from build123d import *

# Parameters (mm, degrees)
SKETCH1_R           = 1.5
BOSS_EXTRUDE1_DEPTH = 1.35
CHAMFER1_SIZE       = 0.4


with BuildPart() as part:
    # Sketch1 → Boss-Extrude1 (new body, symmetric)
    with BuildSketch(Plane(origin=(0, 0, 0), x_dir=(1, 0, 0), z_dir=(0, 1, 0))):
        with BuildLine():
            Line((-13.25, 3.25), (13.25, 3.25))
            ThreePointArc((13.25, 3.25), (16.5, 0), (13.25, -3.25))
            Line((13.25, -3.25), (-13.25, -3.25))
            ThreePointArc((-13.25, -3.25), (-16.5, 0), (-13.25, 3.25))
        make_face()
        with Locations((-13.25, 0)):
            Circle(SKETCH1_R, mode=Mode.SUBTRACT)
        with Locations((13.25, 0)):
            Circle(SKETCH1_R, mode=Mode.SUBTRACT)
        Circle(SKETCH1_R, mode=Mode.SUBTRACT)
    extrude(amount=BOSS_EXTRUDE1_DEPTH, both=True)

    # Chamfer1
    chamfer1_edges = [part.edges().sort_by_distance(p)[0] for p in [
        (16.5, 1.35, 0),
        (0, 1.35, -3.25),
        (-16.5, 1.35, 0),
        (0, 1.35, 3.25),
    ]]
    chamfer(chamfer1_edges, length=CHAMFER1_SIZE)


solid = part.part
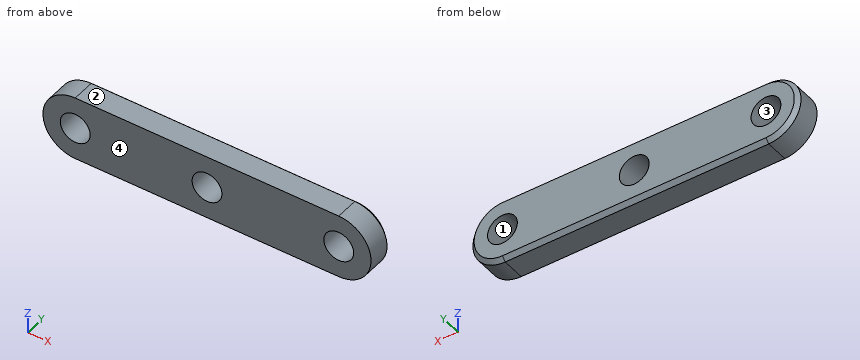
Could you check a few things on this model? Use its own coordinates, in mm. Face numbers are marked on the shaded views. Give positions to 0.01 mm unless a question says otherwise; leave off trailing zeros. Write each loop counter-clockwise with the first axis right and the second up, starting at its lowest first coordinate (ties: lowest second). Pieces come first, ordered by that corner, then holes. Notation, with made-up numbers: (-27, 19.5) -> (-17, 19.5) arc R21 cw to (-17, 50.5) -> close; hole circle Ø7 at (-27.75, 69.25). An arc over 180 degrees is marked (long way). Write each question's results on one line, items separated by ' | '. Start each with the question number.
Q1. Suppose I cut it at A-A, the plane x = 0. List the corners of the cut face in (y, z) for me, and give its area (3 significant figures).
Q2. I need wall thicknesses on probe 1 along X at (y, z) = (0.7, 0); probe 2 along Z at (x, y) = (13.25, -0.5); probe 3 along X at (y, z) = (-0.55, 0.5). Which ranges of each line are inside material? Lowest first, please.
Q3. Suppose I cut it at C-C, the plane z = 1. State how many separate pieces and enclosed holes the cut face has, and give its area (3 significant figures).
Q4. We'd pull the mould along Z, two halves only. Please class the marked faces 1, 2, 3 and 4: +Z half, -Z half, draft (parallel to the pull), parting line (faces both ways), or undercut.
Q5. Suppose I cut it at B-B, the plane y = -0.7. List the corners of the cut face in (x, z) for me, and give its area (3 significant figures).
Q6. I'm going to push a flat-ended pin straight in: pin 1 Ø2.5 at (x, z) = (13.25, 0) entering from -Y. Where does the tip first touch, or does it pass through?
Outcome:
1) outline: (-1.35, -3.25) -> (0.95, -3.25) -> (1.35, -2.85) -> (1.35, -1.5) -> (-1.35, -1.5) -> close; (-1.35, 1.5) -> (1.35, 1.5) -> (1.35, 2.85) -> (0.95, 3.25) -> (-1.35, 3.25) -> close | area: 9.29 mm2
2) probe 1: -16.5 to -14.75, -11.75 to -1.5, 1.5 to 11.75, 14.75 to 16.5 | probe 2: -3.25 to -1.5, 1.5 to 3.25 | probe 3: -16.46 to -14.66, -11.84 to -1.41, 1.41 to 11.84, 14.66 to 16.46
3) separate pieces: 4 | enclosed holes: 0 | area: 70.0 mm2
4) face 1: undercut | face 2: +Z half | face 3: undercut | face 4: draft
5) outline: (-13.25, -3.25) -> (13.25, -3.25) arc R3.25 ccw to (13.25, 3.25) -> (-13.25, 3.25) arc R3.25 ccw to start; hole circle Ø3 at (-13.25, 0); hole circle Ø3 at (0, 0); hole circle Ø3 at (13.25, 0) | area: 184 mm2
6) pin 1: through
